Model file for the job. Use its own axes, mm. A direction names the side the tool comes from. Give positions to 0.01 mm unless a question says otherwise; leave off trailing zeros. Loops run counter-clockwise (first coordinate to the right, second up) from the corner with the lowest first, then second, coordinate; pieces in that order, holes last. Notation, with made-up numbers: M 22,35 L 45,35 A29 cw 45,66 Z; hole C 45,75 d8. An arc over 180 degrees is marked long. Answer in a Markdown table with one row per item.
```python
from build123d import *

# Parameters (mm, degrees)
F0_W      = 180
F0_H      = 110
F1_DEPTH  = 100
F2_W      = 170
F2_H      = 100
F3_DEPTH  = 95
F4_R      = 30
F4_R_2    = 5
F4_R_3    = 10
F5_DEPTH  = 5.001
F6_R      = 6
F8_R      = 4
F6_R_2    = 5
F13_R     = 2
F13_R_2   = 2.5
F18_DEPTH = 20


with BuildPart() as f1:
    # F0 (on Top) → F1 (new body)
    with BuildSketch(Plane.XY):
        Rectangle(F0_W, F0_H)
        with BuildLine():
            Line((-90, 55), (90, 55))
            ThreePointArc((90, 55), (0, 145), (-90, 55))
        make_face()
    extrude(amount=F1_DEPTH)

    # F2 (on face) → F3 (cut)
    with BuildSketch(Plane.XY.offset(100)):
        Rectangle(F2_W, F2_H)
        with BuildLine():
            Line((-85, 50), (85, 50))
            ThreePointArc((85, 50), (0, 140.3125000018), (-85, 50))
        make_face()
    extrude(amount=-F3_DEPTH, mode=Mode.SUBTRACT)

    # F4 (on face) → F5 (cut, through all)
    with BuildSketch(Plane.XY.offset(5)):
        with Locations((0, 90.3125000018)):
            Circle(F4_R)
        with Locations((-55, 0.3125000018)):
            Circle(F4_R_2)
        with Locations((-55, -14.6874999982)):
            Circle(F4_R_2)
        with Locations((55, 0.3125000018)):
            Circle(F4_R_2)
        with Locations((55, -14.6874999982)):
            Circle(F4_R_2)
        with Locations((-50, 20.3125000018)):
            Circle(F4_R_3)
        with Locations((50, 20.3125000018)):
            Circle(F4_R_3)
        with Locations((-55, -29.6874999982)):
            Circle(F4_R_2)
        with Locations((55, -29.6874999982)):
            Circle(F4_R_2)
    extrude(amount=-F5_DEPTH, mode=Mode.SUBTRACT)

    # F6 (on face) → F9 section 0
    with BuildSketch(Plane.XY.offset(5)):
        with Locations((-21.67, 27.6725000018)):
            Circle(F6_R)
    # F8 (on offset) → F9 section 1
    with BuildSketch(Plane.XY.offset(35)):
        with Locations((-21.67, 27.6725000018)):
            Circle(F8_R)
    loft()

    # F6 (on face) → F10 section 0
    with BuildSketch(Plane.XY.offset(5)):
        with Locations((21.67, 27.6725000018)):
            Circle(F6_R)
    # F8 (on offset) → F10 section 1
    with BuildSketch(Plane.XY.offset(35)):
        with Locations((21.67, 27.6725000018)):
            Circle(F8_R)
    loft()

    # F6 (on face) → F11 section 0
    with BuildSketch(Plane.XY.offset(5)):
        with Locations((-23.17, -39.6874999982)):
            Circle(F6_R)
    # F8 (on offset) → F11 section 1
    with BuildSketch(Plane.XY.offset(35)):
        with Locations((-23.17, -39.6874999982)):
            Circle(F8_R)
    loft()

    # F6 (on face) → F12 section 0
    with BuildSketch(Plane.XY.offset(5)):
        with Locations((23.17, -39.6874999982)):
            Circle(F6_R)
    # F8 (on offset) → F12 section 1
    with BuildSketch(Plane.XY.offset(35)):
        with Locations((23.17, -39.6874999982)):
            Circle(F8_R)
    loft()

    # F6 (on face) → F14 section 0
    with BuildSketch(Plane.XY.offset(5)):
        with Locations((27, 117.3125000004)):
            Circle(F6_R_2)
    # F8 (on offset) → F14 section 1
    with BuildSketch(Plane.XY.offset(35)):
        with Locations((27, 117.3125000004)):
            Circle(F8_R)
    loft()

    # F6 (on face) → F15 section 0
    with BuildSketch(Plane.XY.offset(5)):
        with Locations((27, 63.3125000004)):
            Circle(F6_R_2)
    # F8 (on offset) → F15 section 1
    with BuildSketch(Plane.XY.offset(35)):
        with Locations((27, 63.3125000004)):
            Circle(F8_R)
    loft()

    # F6 (on face) → F16 section 0
    with BuildSketch(Plane.XY.offset(5)):
        with Locations((-27, 63.3125000004)):
            Circle(F6_R_2)
    # F8 (on offset) → F16 section 1
    with BuildSketch(Plane.XY.offset(35)):
        with Locations((-27, 63.3125000004)):
            Circle(F8_R)
    loft()

    # F6 (on face) → F17 section 0
    with BuildSketch(Plane.XY.offset(5)):
        with Locations((-27, 117.3125000004)):
            Circle(F6_R_2)
    # F8 (on offset) → F17 section 1
    with BuildSketch(Plane.XY.offset(35)):
        with Locations((-27, 117.3125000004)):
            Circle(F8_R)
    loft()

    # F13 (on face) → F18 (cut)
    with BuildSketch(Plane.XY.offset(35)):
        with Locations((-21.67, 27.6725000018)):
            Circle(F13_R)
        with Locations((21.67, 27.6725000018)):
            Circle(F13_R)
        with Locations((23.17, -39.6874999982)):
            Circle(F13_R)
        with Locations((-23.17, -39.6874999982)):
            Circle(F13_R)
        with Locations((27, 63.3125000004)):
            Circle(F13_R_2)
        with Locations((27, 117.3125000004)):
            Circle(F13_R_2)
        with Locations((-27, 63.3125000004)):
            Circle(F13_R_2)
        with Locations((-27, 117.3125000004)):
            Circle(F13_R_2)
    extrude(amount=-F18_DEPTH, mode=Mode.SUBTRACT)


solid = f1.part
```
Q1. Saw through at C-C (y = 71.5). Give the cut face in (x, z).
Reported:
| item | result |
|---|---|
| outline | M -88.47,0 L -23.37,0 L -23.37,5 L -83.57,5 L -83.57,100 L -88.47,100 Z; M 23.37,0 L 88.47,0 L 88.47,100 L 83.57,100 L 83.57,5 L 23.37,5 Z |
Q2. Probe probe 1 along X at (y, z) = (51, 78); probe 2 along Y at (x, z) = (21.67, 24.5); probe 3 along X at (y, z) = (24, 20.5). List the from-to ranges inside material, lowest first.
Reported:
| item | result |
|---|---|
| probe 1 | -90 to -85.05, 85.05 to 90 |
| probe 2 | -55 to -50, -44.14 to -41.01, -38.36 to -35.23, 22.97 to 25.67, 29.67 to 32.37, 137.51 to 142.35 |
| probe 3 | -90 to -85, -25.01 to -18.33, 18.33 to 25.01, 85 to 90 |
Q3. Mould opens along Y. For faces 3 (the face through (1.98, 144.98, 49.3)), 4 (the face through (21, -41, 35)), 5 (the face through (-1, 24, 0)) say: released by +Y, released by -Y, zero draft, split by the parting line, or undercut.
Reported:
| item | result |
|---|---|
| face 3 | released by +Y |
| face 4 | undercut |
| face 5 | zero draft |
Q4. 3-axis set-ups, long thin cutter, end or side, ignore diameter. For faces 1 (the face through (-30.565, 60.579, 20.21)), 2 (the face through (-59.99, 20.75, 2.54)): which of +Z, -Z, +X, -X, +Y, -Y reach the whole face in a straight line?
Reported:
| item | result |
|---|---|
| face 1 | +Z |
| face 2 | +Z, -Z |
Q5. Saw through at B-B (x = -5.5). Give the cut face in (y, z), and give its area (3 significant figures).
Reported:
| item | result |
|---|---|
| outline | M -55,0 L 60.82,0 L 60.82,5 L -50,5 L -50,100 L -55,100 Z; M 119.8,0 L 144.83,0 L 144.83,100 L 140.13,100 L 140.13,5 L 119.8,5 Z |
| area | 1,630 mm² |
Q6. Drop flat-ended pins along their axis: pin 1 (4 mm diameter, centred on x = -23.5, y = 26, fed in from +Z); pin 2 (3 mm diameter, centred on x = -21.67, y = 27.67, fed in from -Z); pin 3 (3 mm diameter, centred on x = 37.5, y = 111, fed in from +Z); pin 4 (10 mm diameter, centred on y = 70.5, z = 79, fed in from +X). Give the stop position or say it passes through.
Reported:
| item | result |
|---|---|
| pin 1 | z = 35 |
| pin 2 | z = 0 |
| pin 3 | z = 5 |
| pin 4 | x = 89.39 |
Q7. Saw through at A-A (z = 18.5). Give the number of separate pieces and of enclosed holes in the cut face, and give its area (3 significant figures).
Reported:
| item | result |
|---|---|
| separate pieces | 9 |
| enclosed holes | 9 |
| area | 3,710 mm² |
